Check sheet for the modelled part. Datum: model origin and axes. Units: mm. Face numbers are marked on the shaded views. Round coordinates to 2 decimals unless told otherwise and drop trailing zeros. Order: outer loops, then holes, each group sorted by start corner. A loop starts at its lowest first (then second) coordinate and runs counter-clockwise, first axis right, second up. Notation, with made-up numbers: (-1, 2.25) -> (21, 2.25) arc R31 cw to (21, 40.25) -> close; hole circle Ø1 at (26, -24.75). An arc over 180 degrees is marked (long way). Answer in a Markdown table with one row per item. Add a question column.
1. Sectioned sample at A-A, the plane z = -50. Record the boundary of the cut face in (x, y), then the cut area to 3 significant figures.
2. Material ranges on L1, parallel to Y at x = -39.5, z = -41; L2, parallel to Z at x = -55.5, y = -25; L3, parallel to Y at x = -26.5, z = -45, recorded low to high. Write a range as from..to.
3. Draft check along X on the marked faces 1, 2 and 3. Enter one of: +X half, -X half, draft (parallel to the pull), parting line (faces both ways), or undercut.
4. Sectioned sample at D-D, the plane z = -91. Record the boundary of the cut face in (x, y), then the cut area to 3 significant figures.
5. Sectioned sample at C-C, the plane z = -73. Record the boundary of the cut face in (x, y).
6. Sectioned sample at B-B, the plane z = -108. Record the boundary of the cut face in (x, y), then the cut area to 3 significant figures.
7. Depth check by flat-ended pin: P1, Ø12, axis at x = -53.5, y = -21.5, coming from the +Z side; P2, Ø12, axis at y = 9, z = -115.5, coming from the +X side; P3, Ø8, axis at x = -25.7, z = -20, coming from the -Y side; P4, Ø6, axis at x = -36, z = -61.5, coming from the -Y side. Enter the tip coordinate at first touch or a pass-through.
```python
from build123d import *

# Parameters (mm, degrees)
F2_T     = -2.5
F3_W     = 23.2394424225
F3_H     = 43.3458978903
F3_R     = 2.5
F4_DEPTH = 40.0009476822
F5_DEPTH = 40.0009476822


with BuildPart() as f1:
    # F0 (on Front) → F1 (revolve)
    with BuildSketch(Plane.XZ):
        Polygon((-26.3357340748, 0.0224007943), (-26.3357340748, -126.9775992057), (-9.8357340748, -126.9775992057), (12.0191977024, -7.8678405553), (13.5191977024, -7.8678405553), (13.6642136074, -0.0422940365), align=None)
    revolve(axis=Axis((-26.3357340748, 0, -63.4775992057), (0, 0, -1)))

    # F2
    f2_openings = [f1.faces().sort_by_distance(p)[0] for p in [
        (-46.335708, 0, -0.009947),
    ]]
    offset(amount=F2_T, openings=f2_openings, kind=Kind.INTERSECTION)

    # F3 (on Front) → F4 (cut, through all)
    with BuildSketch(Plane.XZ):
        with Locations((-4.2045409791, -108.6729489452)):
            Rectangle(F3_W, F3_H)
        with Locations((-25.6951171905, -20)):
            Circle(F3_R)
    extrude(amount=-F4_DEPTH, mode=Mode.SUBTRACT)

    # F3 (on Front) → F5 (cut, through all)
    with BuildSketch(Plane.XZ):
        with Locations((-4.2045409791, -108.6729489452)):
            Rectangle(F3_W, F3_H)
    extrude(amount=F5_DEPTH, mode=Mode.SUBTRACT)


solid = f1.part
```
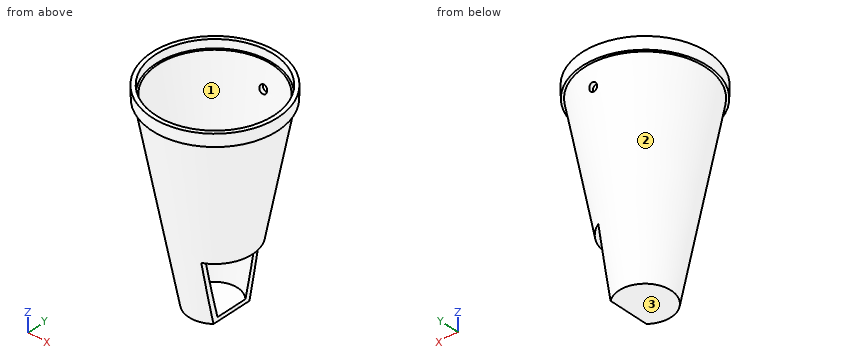
Answer key:
| question | item | result |
|---|---|---|
| 1 | outline | circle Ø61.25 at (-26.34, 0); hole circle Ø56.17 at (-26.34, 0) |
| 1 | area | 469 mm² |
| 2 | L1 | y = -29.47..-26.66, 26.66..29.47 |
| 2 | L2 | z = -7.87..-0.04 |
| 2 | L3 | y = -31.54..-29, 29..31.54 |
| 3 | face 1 | undercut |
| 3 | face 2 | parting line |
| 3 | face 3 | draft |
| 4 | outline | (-15.82, -20.57) -> (-15.82, -17.67) arc R20.56 cw (long way) to (-15.82, 17.67) -> (-15.82, 20.57) arc R23.1 ccw (long way) to start |
| 4 | area | 230 mm² |
| 5 | outline | circle Ø52.81 at (-26.34, 0); hole circle Ø47.72 at (-26.34, 0) |
| 6 | outline | (-15.82, -16.99) -> (-15.82, -13.92) arc R17.44 cw (long way) to (-15.82, 13.92) -> (-15.82, 16.99) arc R19.98 ccw (long way) to start |
| 6 | area | 206 mm² |
| 7 | P1 | stops at z = -0.04 |
| 7 | P2 | stops at x = -15.82 |
| 7 | P3 | stops at y = -36.86 |
| 7 | P4 | stops at y = -27.91 |
